Here's how the part is built. I have some questions about the finished solid (model axes, mm). Face numbers are marked on the shaded views. A direction names the side the tool comes from. Coordinates: 2 decimals unless noted, no trailing zeros. Write each loop counter-clockwise with the first axis right and the second up, starting at its lowest first coordinate (ties: lowest second). Pieces come first, ordered by that corner, then holes. Notation, with made-up numbers: (-3.5, 3.5) -> (23.5, 3.5) arc R23 ccw to (23.5, 20.5) -> close; hole circle Ø1 at (-34, 42). An arc over 180 degrees is marked (long way). Use a Markdown table: item, result. Add a question column.
Item 1: Imagine slicing it at C-C, the plane y = 27.5. Write out the boundary of the cut face in (x, z).
Item 2: Imagine slicing it at B-B, the plane x = 0. Write out the boundary of the cut face in (y, z).
Item 3: Imagine slicing it at A-A, the plane z = 0. Write out the boundary of the cut face in (x, y), and give its area (3 significant figures).
Item 4: If I drill on line 1 along Z through (x, y) = (-3, 5); line 2 along Z through (x, y) = (13, 48); line 3 along X through (y, z) = (25.5, -59.5), over which ranges is the centre line in solid material (lowest first)? Write a range as from..to.
Item 5: Will these pins go through, and if not, where does the flat tip stop? pin 1 Ø8 at (y, z) = (6, -16) entering from +X; pin 2 Ø10 at (y, z) = (19.5, -33) entering from -X; pin 3 Ø12 at (y, z) = (10.5, -33.5) entering from -X; pin 4 Ø2 at (x, y) = (-54.5, 23) entering from -Z.
Item 6: On a 3-axis mill with a long thin cutter (end or side, diameter ignored), from which of +Z, -Z, +X, -X, +Y, -Y can I reach the whole of each face in a straight line? I mean the marked faces 1, 2 and 3. Say none if no direction works.
Item 7: Imagine slicing it at D-D, the plane y = 18.5. Write out the boundary of the cut face in (x, z), and give its area (3 significant figures).
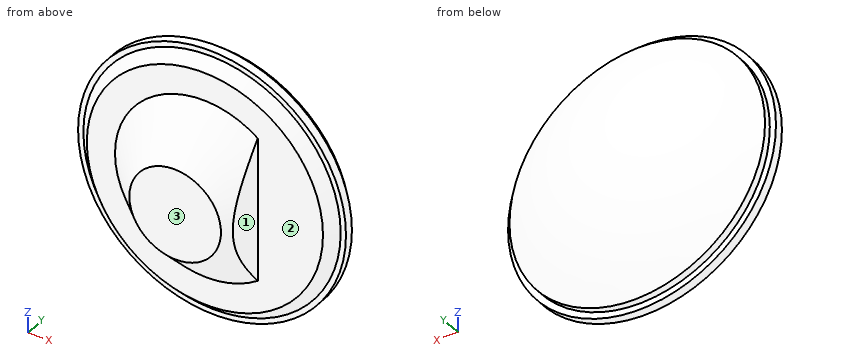
```python
from build123d import *

# Parameters (mm, degrees)
SKETCH2_W          = 70
SKETCH2_H          = 180
CUT_EXTRUDE1_DEPTH = 25


with BuildPart() as part:
    # Sketch1 → Revolve1 (revolve)
    with BuildSketch(Plane.XY, mode=Mode.PRIVATE) as revolve1_sk:
        with BuildLine():
            Line((72.5, 40), (72.5, 36))
            Line((72.5, 36), (76, 36))
            Line((76, 36), (76, 31))
            Line((76, 31), (73, 31))
            Line((73, 31), (67, 25))
            Line((67, 25), (51, 25))
            Line((51, 25), (26, 0))
            Line((26, 0), (0, 0))
            Line((0, 0), (0, 62.2))
            ThreePointArc((0, 62.2), (37.91137692, 56.525667871), (72.5, 40))
        make_face()
    revolve(revolve1_sk.sketch.rotate(Axis((0, 0, 0), (0, -1, 0)), 180), axis=Axis((0, 0, 0), (0, -1, 0)))

    # Sketch2 → Cut-Extrude1 (cut)
    with BuildSketch(Plane.XZ):
        with Locations((65, 0)):
            Rectangle(SKETCH2_W, SKETCH2_H)
    extrude(amount=-CUT_EXTRUDE1_DEPTH, mode=Mode.SUBTRACT)


solid = part.part
```
Ans:
| question | item | result |
|---|---|---|
| 1 | outline | circle Ø139 at (0, 0) |
| 2 | outline | (0, -26) -> (25, -51) -> (25, -67) -> (31, -73) -> (31, -76) -> (36, -76) -> (36, -72.5) -> (40, -72.5) arc R129.48 ccw to (40, 72.5) -> (36, 72.5) -> (36, 76) -> (31, 76) -> (31, 73) -> (25, 67) -> (25, 51) -> (0, 26) -> close |
| 3 | outline | (-76, 31) -> (-73, 31) -> (-67, 25) -> (-51, 25) -> (-26, 0) -> (26, 0) -> (30, 4) -> (30, 25) -> (67, 25) -> (73, 31) -> (76, 31) -> (76, 36) -> (72.5, 36) -> (72.5, 40) arc R129.48 ccw to (-72.5, 40) -> (-72.5, 36) -> (-76, 36) -> close |
| 3 | area | 6,070 mm^2 |
| 4 | line 1 | z = -30.85..30.85 |
| 4 | line 2 | z = -57.5..57.5 |
| 4 | line 3 | x = -31.87..31.87 |
| 5 | pin 1 | stops at x = 30 |
| 5 | pin 2 | stops at x = -39.41 |
| 5 | pin 3 | stops at x = -28.49 |
| 5 | pin 4 | passes through |
| 6 | face 1 | +Z, -Z, +X, -Y |
| 6 | face 2 | -Y |
| 6 | face 3 | +Z, -Z, +X, -X, -Y |
| 7 | outline | (30, -32.87) -> (30, 32.87) arc R44.5 ccw (long way) to start |
| 7 | area | 5,560 mm^2 |
